from build123d import *

# Parameters (mm, degrees)
BOSS_EXTRUDE1_DEPTH = 1.6
SKETCH2_R           = 2.1
CUT_EXTRUDE1_DEPTH  = 2.6
LPATTERN1_COUNT     = 5
LPATTERN1_PITCH     = 8


with BuildPart() as part:
    # Sketch1 → Boss-Extrude1 (new body)
    with BuildSketch(Plane(origin=(0, 0, 0), x_dir=(1, 0, 0), z_dir=(0, 1, 0))):
        with BuildLine():
            Line((4.85, 4.85), (35.15, 4.85))
            ThreePointArc((35.15, 4.85), (40, 0), (35.15, -4.85))
            Line((35.15, -4.85), (4.85, -4.85))
            ThreePointArc((4.85, -4.85), (0, 0), (4.85, 4.85))
        make_face()
    extrude(amount=BOSS_EXTRUDE1_DEPTH)

    # Sketch2 → Cut-Extrude1 (cut, through all)
    with BuildSketch(Plane(origin=(0, 1.6, 0), x_dir=(1, 0, 0), z_dir=(0, 1, 0))):
        with Locations((4, 0)):
            Circle(SKETCH2_R)
    cut_extrude1 = extrude(amount=-CUT_EXTRUDE1_DEPTH, mode=Mode.SUBTRACT)

    # LPattern1: Cut-Extrude1 ×5
    with Locations(*[(i * LPATTERN1_PITCH, 0, 0) for i in range(1, LPATTERN1_COUNT)]):
        add(cut_extrude1, mode=Mode.SUBTRACT)


solid = part.part
Design review of the part built by this model. Coordinates are the model's own, in mm. Give positions to 0.01 mm unless a question says otherwise; leave off trailing zeros. Write each loop counter-clockwise with the first axis right and the second up, starting at its lowest first coordinate (ties: lowest second). Pieces come first, ordered by that corner, then holes. Notation, with made-up numbers: M 21.5,-3.75 L 32.5,-3.75 A26 ccw 32.5,28.25 Z; hole C 40.5,73 d3. An arc over 180 degrees is marked long. Return JSON: item names as keys, results as strings. Group by question number.
Item 1: Take a section at B-B (y = 0.3). Give the boundary of the cut face in (x, z).
Item 2: Wall thickness on line 1 along X through (y, z) = (0.6, 0); line 2 along X through (y, z) = (0.9, 1); line 3 along Z through (x, y) = (28, 1.05): over which ranges is each line inside the solid? List them lowest first.
Item 3: Take a section at C-C (z = -1.25). Give the boundary of the cut face in (x, y).
Item 4: Clearance check with a flat-ended pin moving along its axis: pin 1 Ø5.5 at (x, z) = (4, 0) entering from +Y. State where the tip first meets the part, or that it passes through.
Item 5: Take a section at A-A (x = 12). Give the boundary of the cut face in (y, z), plus the area to 3 significant figures.
Item 6: The part is to be moulded in two halves that separate along Z. For faces 1 (the cylindrical face through (9.9, 0.81, -0.09)), 2 (the flat face through (20, 1, -4.85)), 3 (the flat face through (20, 1.6, 3)), 4 (the cylindrical face through (40, 1, 0)), say which applies: pulls with the +Z half, pulls with the -Z half, needs draft (parallel to the pull), parting line crosses it, or undercut.
Item 7: Take a section at D-D (x = 36). Give the boundary of the cut face in (y, z).
Return value:
{
 "1": {"outline": "M 4.85,-4.85 L 35.15,-4.85 A4.85 ccw 35.15,4.85 L 4.85,4.85 A4.85 ccw Z; hole C 4,0 d4.2; hole C 12,0 d4.2; hole C 20,0 d4.2; hole C 28,0 d4.2; hole C 36,0 d4.2"},
 "2": {"line 1": "x = 0 to 1.9, 6.1 to 9.9, 14.1 to 17.9, 22.1 to 25.9, 30.1 to 33.9, 38.1 to 40", "line 2": "x = 0.1 to 2.15, 5.85 to 10.15, 13.85 to 18.15, 21.85 to 26.15, 29.85 to 34.15, 37.85 to 39.9", "line 3": "z = -4.85 to -2.1, 2.1 to 4.85"},
 "3": {"outline": "M 0.16,0 L 2.31,0 L 2.31,1.6 L 0.16,1.6 Z; M 5.69,0 L 10.31,0 L 10.31,1.6 L 5.69,1.6 Z; M 13.69,0 L 18.31,0 L 18.31,1.6 L 13.69,1.6 Z; M 21.69,0 L 26.31,0 L 26.31,1.6 L 21.69,1.6 Z; M 29.69,0 L 34.31,0 L 34.31,1.6 L 29.69,1.6 Z; M 37.69,0 L 39.84,0 L 39.84,1.6 L 37.69,1.6 Z"},
 "4": {"pin 1": "stops at y = 1.6"},
 "5": {"outline": "M 0,-4.85 L 1.6,-4.85 L 1.6,-2.1 L 0,-2.1 Z; M 0,2.1 L 1.6,2.1 L 1.6,4.85 L 0,4.85 Z", "area": "8.80 mm2"},
 "6": {"face 1": "undercut", "face 2": "pulls with the -Z half", "face 3": "needs draft", "face 4": "parting line crosses it"},
 "7": {"outline": "M 0,-4.77 L 1.6,-4.77 L 1.6,-2.1 L 0,-2.1 Z; M 0,2.1 L 1.6,2.1 L 1.6,4.77 L 0,4.77 Z"}
}
